Here's how the part is built. I have some questions about the finished solid (model axes, mm). A direction names the side the tool comes from. Give positions to 0.01 mm unless a question says otherwise; leave off trailing zeros. Loops run counter-clockwise (first coordinate to the right, second up) from the corner with the lowest first, then second, coordinate; pieces in that order, holes last. Notation, with made-up numbers: (-16.75, -13.5) - (11.25, -13.5) arc R27 ccw to (11.25, 4.5) - close; hole circle Ø8 at (69, -24.5). An arc over 180 degrees is marked (long way). Use a Markdown table: item, result.
from build123d import *

# Parameters (mm, degrees)
RESSALTO_EXTRUS_O1_DEPTH = 5
CORTE_EXTRUS_O1_DEPTH    = 5
ESBO_O4_R                = 1.5
CORTE_EXTRUS_O2_DEPTH    = 10
ESBO_O6_W                = 8
ESBO_O6_H                = 5
CORTE_EXTRUS_O3_DEPTH    = 5
CORTE_EXTRUS_O4_DEPTH    = 10
ESBO_O9_W                = 8
ESBO_O9_H                = 5
CORTE_EXTRUS_O5_DEPTH    = 5


with BuildPart() as part:
    # Esboço1 → Ressalto-extrusão1 (new body)
    with BuildSketch(Plane(origin=(0, 0, 0), x_dir=(1, 0, 0), z_dir=(0, 1, 0))):
        with BuildLine():
            Line((-43.336132643, 103.024644241), (66.663867357, 103.024644241))
            ThreePointArc((66.663867357, 103.024644241), (73.734935168, 100.095712053), (76.663867357, 93.024644241))
            Line((76.663867357, 93.024644241), (76.663867357, -26.975355759))
            ThreePointArc((76.663867357, -26.975355759), (73.734935168, -34.046423571), (66.663867357, -36.975355759))
            Line((66.663867357, -36.975355759), (-43.336132643, -36.975355759))
            ThreePointArc((-43.336132643, -36.975355759), (-50.407200455, -34.046423571), (-53.336132643, -26.975355759))
            Line((-53.336132643, -26.975355759), (-53.336132643, 93.024644241))
            ThreePointArc((-53.336132643, 93.024644241), (-50.407200455, 100.095712053), (-43.336132643, 103.024644241))
        make_face()
    extrude(amount=RESSALTO_EXTRUS_O1_DEPTH)

    # Esboço2 → Corte-extrusão1 (cut)
    with BuildSketch(Plane(origin=(0, 5, 0), x_dir=(1, 0, 0), z_dir=(0, 1, 0))):
        with BuildLine():
            Line((-42.336132643, 94.024644241), (-21.336132643, 94.024644241))
            ThreePointArc((-21.336132643, 94.024644241), (-19.921919081, 93.438857803), (-19.336132643, 92.024644241))
            Line((-19.336132643, 92.024644241), (-19.336132643, 51.024644241))
            ThreePointArc((-19.336132643, 51.024644241), (-19.921919081, 49.610430679), (-21.336132643, 49.024644241))
            Line((-21.336132643, 49.024644241), (-42.336132643, 49.024644241))
            ThreePointArc((-42.336132643, 49.024644241), (-43.750346206, 49.610430679), (-44.336132643, 51.024644241))
            Line((-44.336132643, 51.024644241), (-44.336132643, 92.024644241))
            ThreePointArc((-44.336132643, 92.024644241), (-43.750346206, 93.438857803), (-42.336132643, 94.024644241))
        make_face()
        with BuildLine():
            Line((44.663867357, 94.024644241), (65.663867357, 94.024644241))
            ThreePointArc((65.663867357, 94.024644241), (67.078080919, 93.438857803), (67.663867357, 92.024644241))
            Line((67.663867357, 92.024644241), (67.663867357, 51.024644241))
            ThreePointArc((67.663867357, 51.024644241), (67.078080919, 49.610430679), (65.663867357, 49.024644241))
            Line((65.663867357, 49.024644241), (44.663867357, 49.024644241))
            ThreePointArc((44.663867357, 49.024644241), (43.249653794, 49.610430679), (42.663867357, 51.024644241))
            Line((42.663867357, 51.024644241), (42.663867357, 92.024644241))
            ThreePointArc((42.663867357, 92.024644241), (43.249653794, 93.438857803), (44.663867357, 94.024644241))
        make_face()
    extrude(amount=-CORTE_EXTRUS_O1_DEPTH, mode=Mode.SUBTRACT)

    # Esboço4 → Corte-extrusão2 (cut)
    with BuildSketch(Plane(origin=(0, 5, 0), x_dir=(1, 0, 0), z_dir=(0, 1, 0))):
        with Locations(Location((-7.836132643, 59.524644241, 0), (0, 0, 270))):
            Circle(ESBO_O4_R)
        with Locations(Location((31.163867357, 59.524644241, 0), (0, 0, 270))):
            Circle(ESBO_O4_R)
        with Locations(Location((-7.836132643, 83.524644241, 0), (0, 0, 270))):
            Circle(ESBO_O4_R)
        with Locations(Location((31.163867357, 83.524644241, 0), (0, 0, 270))):
            Circle(ESBO_O4_R)
    extrude(amount=-CORTE_EXTRUS_O2_DEPTH, mode=Mode.SUBTRACT)

    # Esboço6 → Corte-extrusão3 (cut)
    with BuildSketch(Plane.ZY.offset(53.336132643)):
        with Locations((16.975355759, 2.5)):
            Rectangle(ESBO_O6_W, ESBO_O6_H)
    extrude(amount=-CORTE_EXTRUS_O3_DEPTH, mode=Mode.SUBTRACT)

    # Esboço7 → Corte-extrusão4 (cut)
    with BuildSketch(Plane.XZ):
        with BuildLine():
            Line((18.663867357, -77.524644241), (4.663867357, -77.524644241))
            ThreePointArc((4.663867357, -77.524644241), (3.249653794, -76.938857803), (2.663867357, -75.524644241))
            Line((2.663867357, -75.524644241), (2.663867357, -67.524644241))
            ThreePointArc((2.663867357, -67.524644241), (3.249653794, -66.110430679), (4.663867357, -65.524644241))
            Line((4.663867357, -65.524644241), (18.663867357, -65.524644241))
            ThreePointArc((18.663867357, -65.524644241), (20.078080919, -66.110430679), (20.663867357, -67.524644241))
            Line((20.663867357, -67.524644241), (20.663867357, -75.524644241))
            ThreePointArc((20.663867357, -75.524644241), (20.078080919, -76.938857803), (18.663867357, -77.524644241))
        make_face()
    extrude(amount=-CORTE_EXTRUS_O4_DEPTH, mode=Mode.SUBTRACT)

    # Esboço9 → Corte-extrusão5 (cut)
    with BuildSketch(Plane(origin=(76.663867357, 0, 0), x_dir=(0, 0, -1), z_dir=(1, 0, 0))):
        with Locations((-16.975355759, 2.5)):
            Rectangle(ESBO_O9_W, ESBO_O9_H)
    extrude(amount=-CORTE_EXTRUS_O5_DEPTH, mode=Mode.SUBTRACT)


solid = part.part
(1) On a 3-axis mill with a long thin cutter (end or side, diameter ignored), from which of +Z, -Z, +X, -X, +Y, -Y can I reach the whole of each face in a straight line? I mean faces 1 (the face through (-51, 2, 20.975)), 2 (the face through (13, 5, -34)), 3 (the face through (-53.336, 2, 24)), 4 (the face through (74, 2, 20.975)), 5 (the face through (-32, 3, -94.025)). Say none if no direction works.
A:
| item | result |
|---|---|
| face 1 | -X, +Y, -Y |
| face 2 | +Z, -Z, +X, -X, +Y |
| face 3 | +Z, -Z, -X, +Y, -Y |
| face 4 | +X, +Y, -Y |
| face 5 | +Y, -Y |
(2) If I drill on line 1 (Z direction, x = 31, y = 3.25); line 2 (X direction, y = 3.65, z = -56); line 3 (Z direction, x = 16, y = 1.5), over which ranges is the centre line in solid material (lowest first)?
A:
| item | result |
|---|---|
| line 1 | -103.02 to -85.02, -82.03 to -61.02, -58.03 to 36.98 |
| line 2 | -53.34 to -44.34, -19.34 to 42.66, 67.66 to 76.66 |
| line 3 | -103.02 to -77.52, -65.52 to 36.98 |
(3) We'd pull the mould along Z, two halves only. Please class faces 6 (the face through (76.664, 2, -41)), 7 (the face through (2.664, 2, -72)), 8 (the face through (-32, 3, -49.025)), 9 (the face through (12, 2, 36.975)): pulls with the +Z half, pulls with the -Z half, needs draft (parallel to the pull), parting line crosses it, or undercut.
A:
| item | result |
|---|---|
| face 6 | needs draft |
| face 7 | undercut |
| face 8 | undercut |
| face 9 | pulls with the +Z half |
(4) Suppose I cut it at A-A on x = -30. Write out the boundary of the cut face in (y, z), plus the area to 3 significant figures.
A:
| item | result |
|---|---|
| outline | (0, -103.02) - (5, -103.02) - (5, -94.02) - (0, -94.02) - close; (0, -49.02) - (5, -49.02) - (5, 36.98) - (0, 36.98) - close |
| area | 475 mm2 |
(5) Will these pins go through, and if not, where does the flat tip stop? pin 1 (3 mm diameter, centred on x = 25, z = -24, fed in from -Y); pin 2 (2.5 mm diameter, centred on y = 2.5, z = 18, fed in from -X).
A:
| item | result |
|---|---|
| pin 1 | y = 0 |
| pin 2 | x = -48.34 |
(6) Suppose I cut it at B-B on y = 1.95. Count the separate pieces of the cut face and the enclosed holes in it, plus the area to 3 significant figures.
A:
| item | result |
|---|---|
| separate pieces | 1 |
| enclosed holes | 7 |
| area | 15,600 mm2 |
